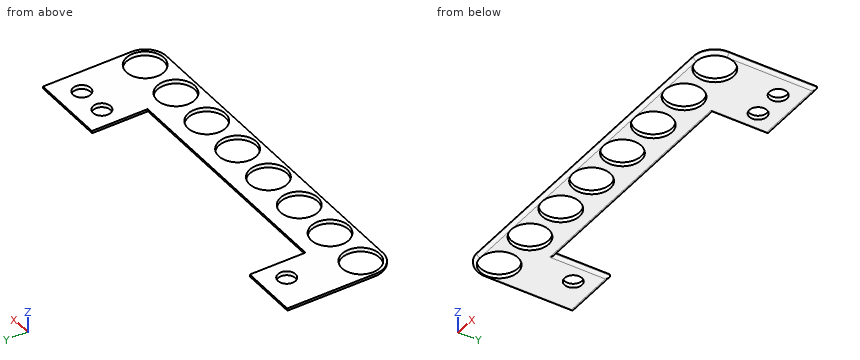
from build123d import *

# Parameters (mm, degrees)
F0_R        = 3.2
F0_R_2      = 1.5
F1_DEPTH    = 0.7
F2_R        = 0.49999
F3_T1_DEPTH = 9.7
F3_T4_ANGLE = 90
F3_T6_ANGLE = 90


# Not quite as in the source:
# - a fillet or chamfer that OpenCascade refuses, or shapes differently, is made with other operations: its cross-section is extruded or revolved along the edge and cut away or added
# - a fillet or chamfer is up to 0.001 mm smaller than in the source, because OpenCascade refuses the exact size


with BuildPart() as f1:
    # F0 (on Top) → F1 (new body)
    with BuildSketch(Plane.XY):
        Polygon((-22, 18.7), (-31.7, 18.7), (-31.7, 0), (-18.3513443917, 0), (-10.3513443917, 0), (31.7, 0), (31.7, 18.7), (19, 18.7), (19, 9.2), (-22, 9.2), align=None)
        with Locations((-28, 3.7)):
            Circle(F0_R, mode=Mode.SUBTRACT)
        with Locations((-20, 3.7)):
            Circle(F0_R, mode=Mode.SUBTRACT)
        with Locations((-12, 3.7)):
            Circle(F0_R, mode=Mode.SUBTRACT)
        with Locations((-4, 3.7)):
            Circle(F0_R, mode=Mode.SUBTRACT)
        with Locations((4, 3.7)):
            Circle(F0_R, mode=Mode.SUBTRACT)
        with Locations((12, 3.7)):
            Circle(F0_R, mode=Mode.SUBTRACT)
        with Locations((20, 3.7)):
            Circle(F0_R, mode=Mode.SUBTRACT)
        with Locations((28, 3.7)):
            Circle(F0_R, mode=Mode.SUBTRACT)
        with Locations((-25.5, 14.7)):
            Circle(F0_R_2, mode=Mode.SUBTRACT)
        with Locations((22.5, 14.7)):
            Circle(F0_R_2, mode=Mode.SUBTRACT)
        with Locations((27.7, 14.7)):
            Circle(F0_R_2, mode=Mode.SUBTRACT)
    extrude(amount=F1_DEPTH)

    # F2 (radius 0.5 in the source; OpenCascade refuses exactly that, so slightly less here)
    f2_edges = [f1.edges().sort_by_distance(p)[0] for p in [
        (-31.7, 9.35, 0),
        (0, 0, 0),
        (31.7, 9.35, 0),
        (25.35, 18.7, 0),
        (19, 13.95, 0),
        (-1.5, 9.2, 0),
        (-22, 13.95, 0),
        (-26.85, 18.7, 0),
    ]]
    fillet(f2_edges, radius=F2_R)

    # F3: fillet of radius 3.6 on 4 edges, made by hand

    # F3_s2 → F3_t1 (cut)
    with BuildSketch(Plane.XY):
        with BuildLine():
            ThreePointArc((-28.1, 0), (-30.6455844123, 1.0544155877), (-31.7, 3.6))
            Line((-31.7, 3.6), (-31.7, 0))
            Line((-31.7, 0), (-28.1, 0))
        make_face()
        with BuildLine():
            ThreePointArc((28.1, 0), (30.6455844123, 1.0544155877), (31.7, 3.6))
            Line((31.7, 3.6), (31.7, 0))
            Line((31.7, 0), (28.1, 0))
        make_face()
    extrude(amount=F3_T1_DEPTH, mode=Mode.SUBTRACT)

    # F3_s3 → F3_t4 (revolve, cut)
    with BuildSketch(Plane.YZ.offset(-28.1)):
        with BuildLine():
            ThreePointArc((0.49999, 0), (0.1464436805, 0.1464436805), (0, 0.49999))
            Line((0, 0.49999), (0, 0))
            Line((0, 0), (0.49999, 0))
        make_face()
    revolve(axis=Axis((-28.1, 3.6, 0), (0, 0, -1)), revolution_arc=F3_T4_ANGLE, mode=Mode.SUBTRACT)

    # F3_s5 → F3_t6 (revolve, cut)
    with BuildSketch(Plane.XZ.offset(-3.6)):
        with BuildLine():
            ThreePointArc((31.20001, 0), (31.5535563195, 0.1464436805), (31.7, 0.49999))
            Line((31.7, 0.49999), (31.7, 0))
            Line((31.7, 0), (31.20001, 0))
        make_face()
    revolve(axis=Axis((28.1, 3.6, 0), (0, 0, -1)), revolution_arc=F3_T6_ANGLE, mode=Mode.SUBTRACT)


solid = f1.part
The model under review builds one solid part; all positions refer to its coordinate system, in mm. Round coordinates to 2 decimals unless told otherwise and drop trailing zeros. Loops run counter-clockwise (first coordinate to the right, second up) from the corner with the lowest first, then second, coordinate; pieces in that order, holes last. Notation, with made-up numbers: M 73,25.5 L 98,25.5 A17 ccw 98,41.5 Z; hole C 68,62 d8. An arc over 180 degrees is marked long. Answer as a JSON object with one key per item and string values.
Item 1: We need section A-A, the plane y = 10.75. State the section outline as (x, z) points.
Check sheet entries:
{"outline": "M -31.7,0.5 A0.5 ccw -31.2,0 L -22.5,0 A0.5 ccw -22,0.5 L -22,0.7 L -31.7,0.7 Z; M 19,0.5 A0.5 ccw 19.5,0 L 31.2,0 A0.5 ccw 31.7,0.5 L 31.7,0.7 L 19,0.7 Z"}
Item 2: We need section D-D, the plane z = 0.3. State how many separate pieces and enclosed holes the cut face has, and give its area (3 significant figures).
Check sheet entries:
{"separate pieces": "1", "enclosed holes": "11", "area": "504 mm2"}
Item 3: For line 1 along X through (y, z) = (15.75, 0.2); line 2 along Y through (x, z) = (4, 0.5); line 3 along X through (y, z) = (10, 0.65), list the stretches that pass through material, from the lowest coordinate up.
Check sheet entries:
{"line 1": "-31.6 to -26.57, -24.43 to -22.1, 19.1 to 21.43, 23.57 to 26.63, 28.77 to 31.6", "line 2": "0 to 0.5, 6.9 to 9.2", "line 3": "-31.7 to -22, 19 to 31.7"}
Item 4: We need section C-C, the plane x = -25.5. State the section outline as (y, z) points, and give its area (3 significant figures).
Check sheet entries:
{"outline": "M 0,0.5 A0.5 ccw 0.5,0 L 1.7,0 L 1.7,0.7 L 0,0.7 Z; M 5.7,0 L 13.2,0 L 13.2,0.7 L 5.7,0.7 Z; M 16.2,0 L 18.2,0 A0.5 ccw 18.7,0.5 L 18.7,0.7 L 16.2,0.7 Z", "area": "8.09 mm2"}
